```python
from build123d import *

# Parameters (mm, degrees)
SKETCH1_R           = 13
BOSS_EXTRUDE1_DEPTH = 50
SKETCH2_R           = 15
BOSS_EXTRUDE2_DEPTH = 28
SKETCH3_R           = 2.5
BOSS_EXTRUDE3_DEPTH = 13
SKETCH4_W           = 2
SKETCH4_H           = 4
CUT_EXTRUDE1_DEPTH  = 13


with BuildPart() as part:
    # Sketch1 → Boss-Extrude1 (new body)
    with BuildSketch(Plane.XY):
        Circle(SKETCH1_R)
    extrude(amount=BOSS_EXTRUDE1_DEPTH)

    # Sketch2 → Boss-Extrude2 (add)
    with BuildSketch(Plane.XY.offset(50)):
        Circle(SKETCH2_R)
    extrude(amount=BOSS_EXTRUDE2_DEPTH)

    # Sketch3 → Boss-Extrude3 (add)
    with BuildSketch(Plane.XY.offset(78)):
        with Locations(Location((0, -7.5, 0), (0, 0, 180))):
            Circle(SKETCH3_R)
    extrude(amount=BOSS_EXTRUDE3_DEPTH)

    # Sketch4 → Cut-Extrude1 (cut)
    with BuildSketch(Plane.XY.offset(91)):
        with Locations((-2.5, -7.5)):
            Rectangle(SKETCH4_W, SKETCH4_H)
    extrude(amount=-CUT_EXTRUDE1_DEPTH, mode=Mode.SUBTRACT)


solid = part.part
```
Can you work these out from the model? Positions are in its coordinate system, mm. A direction names the side the tool comes from. Coordinates: 2 decimals unless noted, no trailing zeros. Loops run counter-clockwise (first coordinate to the right, second up) from the corner with the lowest first, then second, coordinate; pieces in that order, holes last. Notation, with made-up numbers: M -27,-20.75 L -11,-20.75 A19 cw -11,-7.75 Z; hole C -27.75,55 d7. An arc over 180 degrees is marked long. Put each result on its own line as item: value. Start each with the question number.
(1) Imagine slicing it at C-C on z = 47. List the corners of the cut face in (x, y) for me.
(2) Which directions (+Z, -Z, +X, -X, +Y, -Y) give clear straight access to the entire face, cutting with the end or side of a thin tool? Please do faces 1 (the face through (-14.985, 0.66, 63.804)), 2 (the face through (-0.1, 13.4, 50)), 3 (the face through (-1.5, -8, 85)), 4 (the face through (2.5, -7.6, 84.4)).
(3) Imagine slicing it at B-B on y = 0. List the corners of the cut face in (x, z) for me, and give its area (3 significant figures).
(4) Imagine slicing it at A-A on x = 0. List the corners of the cut face in (y, z) for me, and give its area (4 significant figures).
(5) I need wall thicknesses on probe 1 along Z at (x, y) = (5, -2.5); probe 2 along X at (y, z) = (-10.5, 52.5); probe 3 along Y at (x, z) = (-8.25, 76). Which ranges of each line are inside material? Lowest first, please.
(6) Imagine slicing it at D-D on x = -9.25. List the corners of the cut face in (y, z) for me.
(7) Will these pins go through, and if not, where does the flat tip stop? pin 1 Ø1 at (y, z) = (11, 55) entering from -X; pin 2 Ø3 at (x, y) = (1, 7) entering from +Z; pin 3 Ø1 at (y, z) = (-1.5, 27) entering from +X.
Worked answers:
1. outline: C 0,0 d26
2. face 1: +Z, -Z
2. face 2: -Z
2. face 3: +Z, -X, +Y, -Y
2. face 4: +Z
3. outline: M -15,50 L -13,50 L -13,0 L 13,0 L 13,50 L 15,50 L 15,78 L -15,78 Z
3. area: 2,140 mm2
4. outline: M -15,50 L -13,50 L -13,0 L 13,0 L 13,50 L 15,50 L 15,78 L -5,78 L -5,91 L -10,91 L -10,78 L -15,78 Z
4. area: 2,205 mm2
5. probe 1: z = 0 to 78
5. probe 2: x = -10.71 to 10.71
5. probe 3: y = -12.53 to 12.53
6. outline: M -11.81,50 L -9.13,50 L -9.13,0 L 9.13,0 L 9.13,50 L 11.81,50 L 11.81,78 L -11.81,78 Z
7. pin 1: stops at x = -10.71
7. pin 2: stops at z = 78
7. pin 3: stops at x = 12.96
